```python
from build123d import *

# Parameters (mm, degrees)
SKETCH1_W                     = 97
SKETCH1_H                     = 60
BASE_DEPTH                    = 6
SKETCH2_R                     = 12
STEPPERCASEHOLE_DEPTH         = 7
FILLETEDGES3MM_R              = 3
F_3_5MM_CABLETIEHOLES_D       = 3.5
F_5_2_5_2_HOLESFORCORNERS_D   = 5.2
F_3_5_3_5_STEPPERMOUNTHOLES_D = 3.5


with BuildPart() as part:
    # Sketch1 → Base (new body)
    with BuildSketch(Plane(origin=(0, 0, 0), x_dir=(1, 0, 0), z_dir=(0, 1, 0))):
        Rectangle(SKETCH1_W, SKETCH1_H)
    extrude(amount=BASE_DEPTH)

    # Sketch2 → StepperCaseHole (cut, through all)
    with BuildSketch(Plane(origin=(0, 6, 0), x_dir=(1, 0, 0), z_dir=(0, 1, 0))):
        with Locations((0, 5)):
            Circle(SKETCH2_R)
    extrude(amount=-STEPPERCASEHOLE_DEPTH, mode=Mode.SUBTRACT)

    # FilletEdges3mm
    filletedges3mm_edges = [part.edges().sort_by_distance(p)[0] for p in [
        (-48.5, 3, -30),
        (48.5, 3, -30),
        (48.5, 3, 30),
        (-48.5, 3, 30),
    ]]
    fillet(filletedges3mm_edges, radius=FILLETEDGES3MM_R)

    # Ø3.5mm CableTieHoles (through all)
    with Locations(Plane(origin=(0, 0, 0), x_dir=(-1, 0, 0), z_dir=(0, -1, 0))):
        with Locations((-44, 25.5), (44, 25.5)):
            Hole(F_3_5MM_CABLETIEHOLES_D / 2)

    # Ø5.2 (5.2) HolesForCorners (through all)
    with Locations(Plane(origin=(0, 6, 0), x_dir=(1, 0, 0), z_dir=(0, 1, 0))):
        with Locations((-40, 0), (-40, -20), (40, 0), (40, -20)):
            Hole(F_5_2_5_2_HOLESFORCORNERS_D / 2)

    # Ø3.5 (3.5) StepperMountHoles (through all)
    with Locations(Plane(origin=(0, 6, 0), x_dir=(1, 0, 0), z_dir=(0, 1, 0))):
        with Locations((-15.5, 20.5), (-15.5, -10.5), (15.5, -10.5), (15.5, 20.5)):
            Hole(F_3_5_3_5_STEPPERMOUNTHOLES_D / 2)


solid = part.part
```
Here's how the part is built. I have some questions about the finished solid (model axes, mm). Coordinates: 2 decimals unless noted, no trailing zeros. Order: outer loops, then holes, each group sorted by start corner. A loop starts at its lowest first (then second) coordinate and runs counter-clockwise, first axis right, second up.
1) I need wall thicknesses on line 1 (Z direction, x = -15.5, y = 4.5); line 2 (X direction, y = 3.75, z = -20.5); line 3 (Z direction, x = -44, y = 3.6). Which ranges of each line are inside material? Lowest first, please.
2) We'd pull the mould along X, two halves only. Please class faces 1 (the face through (-47.64, 3.04, 29.1)), 2 (the face through (-11.99, 3.04, -5.53)), 3 (the face through (-1, 3, -30)), 4 (the face through (42.6, 3, 19.9)): +X half, -X half, draft (parallel to the pull), parting line (faces both ways), or undercut.
3) Imagine slicing it at D-D on z = -5. List the corners of the cut face in (x, y) for me, and give its area (3 significant figures).
4) Imagine slicing it at B-B on y = 3.25. State how many separate pieces and enclosed holes the cut face has, and give its area (3 significant figures).
5) Imagine slicing it at A-A on x = 15.5. List the corners of the cut face in (y, z) for me, and give its area (3 significant figures).
6) Imagine slicing it at C-C on x = 44. List the corners of the cut face in (y, z) for me.
Response values:
1. line 1: z = -30 to -22.25, -18.75 to 8.75, 12.25 to 30
1. line 2: x = -48.5 to -17.25, -13.75 to 13.75, 17.25 to 48.5
1. line 3: z = -30 to -27.25, -23.75 to 30
2. face 1: -X half
2. face 2: undercut
2. face 3: draft
2. face 4: undercut
3. outline: (-48.5, 0) - (-12, 0) - (-12, 6) - (-48.5, 6) - close; (12, 0) - (48.5, 0) - (48.5, 6) - (12, 6) - close
3. area: 438 mm2
4. separate pieces: 1
4. enclosed holes: 11
4. area: 5,220 mm2
5. outline: (0, -30) - (6, -30) - (6, -22.25) - (0, -22.25) - close; (0, -18.75) - (6, -18.75) - (6, 8.75) - (0, 8.75) - close; (0, 12.25) - (6, 12.25) - (6, 30) - (0, 30) - close
5. area: 318 mm2
6. outline: (0, -30) - (6, -30) - (6, -27.25) - (0, -27.25) - close; (0, -23.75) - (6, -23.75) - (6, 30) - (0, 30) - close
